from build123d import *

# Parameters (mm, degrees)
ESBO_O1_W                = 514
ESBO_O1_H                = 507
RESSALTO_EXTRUS_O1_DEPTH = 5
ESBO_O2_W                = 5
ESBO_O2_H                = 253.5
RESSALTO_EXTRUS_O2_DEPTH = 10
ESBO_O6_W                = 5
ESBO_O6_H                = 253.5
RESSALTO_EXTRUS_O3_DEPTH = 10
ESBO_O7_W                = 3
ESBO_O7_H                = 253.5
CORTE_EXTRUS_O1_DEPTH    = 10
ESBO_O9_W                = 3
ESBO_O9_H                = 253.5
CORTE_EXTRUS_O3_DEPTH    = 10
ESBO_O10_W               = 514
ESBO_O10_H               = 5
RESSALTO_EXTRUS_O4_DEPTH = 10
ESBO_O15_W               = 512
ESBO_O15_H               = 3
CORTE_EXTRUS_O11_DEPTH   = 10
ESBO_O16_W               = 3
ESBO_O16_H               = 1
CORTE_EXTRUS_O12_DEPTH   = 10
ESBO_O20_R               = 15
RESSALTO_EXTRUS_O5_DEPTH = 10
ESBO_O21_W               = 1
ESBO_O21_H               = 29
CORTE_EXTRUS_O13_DEPTH   = 10


with BuildPart() as part:
    # Esboço1 → Ressalto-extrusão1 (new body)
    with BuildSketch(Plane(origin=(0, 0, 0), x_dir=(1, 0, 0), z_dir=(0, 1, 0))):
        with Locations((159.395426849, -182.414405214)):
            Rectangle(ESBO_O1_W, ESBO_O1_H)
    extrude(amount=RESSALTO_EXTRUS_O1_DEPTH)

    # Esboço2 → Ressalto-extrusão2 (add)
    with BuildSketch(Plane(origin=(0, 5, 0), x_dir=(1, 0, 0), z_dir=(0, 1, 0))):
        with Locations((-95.104573151, -55.664405214)):
            Rectangle(ESBO_O2_W, ESBO_O2_H)
    extrude(amount=RESSALTO_EXTRUS_O2_DEPTH)

    # Esboço6 → Ressalto-extrusão3 (add)
    with BuildSketch(Plane(origin=(0, 5, 0), x_dir=(1, 0, 0), z_dir=(0, 1, 0))):
        with Locations((413.895426849, -55.664405214)):
            Rectangle(ESBO_O6_W, ESBO_O6_H)
    extrude(amount=RESSALTO_EXTRUS_O3_DEPTH)

    # Esboço7 → Corte-extrusão1 (cut)
    with BuildSketch(Plane(origin=(0, 15, 0), x_dir=(1, 0, 0), z_dir=(0, 1, 0))):
        with Locations((-95.104573151, -55.664405214)):
            Rectangle(ESBO_O7_W, ESBO_O7_H)
    extrude(amount=-CORTE_EXTRUS_O1_DEPTH, mode=Mode.SUBTRACT)

    # Esboço9 → Corte-extrusão3 (cut)
    with BuildSketch(Plane(origin=(0, 15, 0), x_dir=(1, 0, 0), z_dir=(0, 1, 0))):
        with Locations((413.895426849, -55.664405214)):
            Rectangle(ESBO_O9_W, ESBO_O9_H)
    extrude(amount=-CORTE_EXTRUS_O3_DEPTH, mode=Mode.SUBTRACT)

    # Esboço10 → Ressalto-extrusão4 (add)
    with BuildSketch(Plane(origin=(0, 5, 0), x_dir=(1, 0, 0), z_dir=(0, 1, 0))):
        with Locations((159.395426849, 68.585594786)):
            Rectangle(ESBO_O10_W, ESBO_O10_H)
    extrude(amount=RESSALTO_EXTRUS_O4_DEPTH)

    # Esboço15 → Corte-extrusão11 (cut)
    with BuildSketch(Plane(origin=(0, 15, 0), x_dir=(1, 0, 0), z_dir=(0, 1, 0))):
        with Locations((159.395426849, 68.585594786)):
            Rectangle(ESBO_O15_W, ESBO_O15_H)
    extrude(amount=-CORTE_EXTRUS_O11_DEPTH, mode=Mode.SUBTRACT)

    # Esboço16 → Corte-extrusão12 (cut)
    with BuildSketch(Plane(origin=(0, 15, 0), x_dir=(1, 0, 0), z_dir=(0, 1, 0))):
        with Locations((413.895426849, 66.585594786)):
            Rectangle(ESBO_O16_W, ESBO_O16_H)
        with Locations((-95.104573151, 66.585594786)):
            Rectangle(ESBO_O16_W, ESBO_O16_H)
    extrude(amount=-CORTE_EXTRUS_O12_DEPTH, mode=Mode.SUBTRACT)

    # Esboço20 → Ressalto-extrusão5 (add)
    with BuildSketch(Plane.XZ):
        with Locations(Location((-47.604573151, 385.914405214, 0), (0, 0, 90))):
            Circle(ESBO_O20_R)
        with Locations(Location((366.395426849, 385.914405214, 0), (0, 0, 90))):
            Circle(ESBO_O20_R)
        with Locations(Location((366.395426849, -21.085594786, 0), (0, 0, 90))):
            Circle(ESBO_O20_R)
        with Locations(Location((-47.604573151, -21.085594786, 0), (0, 0, 90))):
            Circle(ESBO_O20_R)
    extrude(amount=RESSALTO_EXTRUS_O5_DEPTH)

    # Esboço21 → Corte-extrusão13 (cut)
    with BuildSketch(Plane(origin=(0, 15, 0), x_dir=(1, 0, 0), z_dir=(0, 1, 0))):
        with Locations((411.895426849, 51.585594786)):
            Rectangle(ESBO_O21_W, ESBO_O21_H)
        with Locations((415.895426849, 51.585594786)):
            Rectangle(ESBO_O21_W, ESBO_O21_H)
    extrude(amount=-CORTE_EXTRUS_O13_DEPTH, mode=Mode.SUBTRACT)


solid = part.part
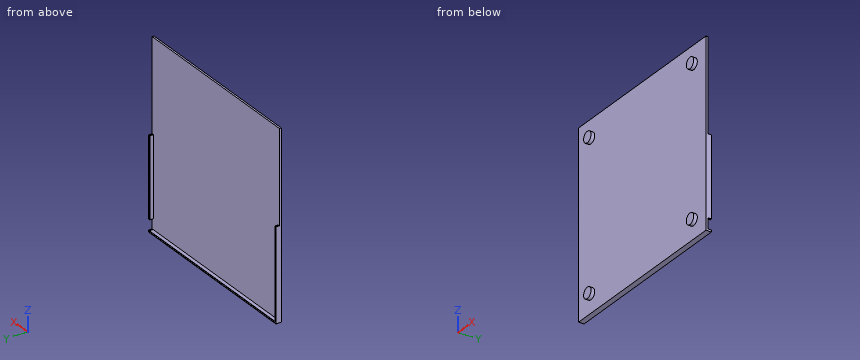
Verification items for the finished model (mm, model axes). Round coordinates to 2 decimals unless told otherwise and drop trailing zeros. Order: outer loops, then holes, each group sorted by start corner. A loop starts at its lowest first (then second) coordinate and runs counter-clockwise, first axis right, second up.
1. Section check D-D on z = 232. Record the cut outline in (x, y), then the cut area to 3 significant figures.
Final values:
outline: (-97.6, 0) - (416.4, 0) - (416.4, 5) - (-97.6, 5) - close
area: 2,570 mm2
2. Section check A-A on x = 321. Record the cut outline in (y, z).
Final values:
outline: (0, -71.09) - (15, -71.09) - (15, -70.09) - (5, -70.09) - (5, -67.09) - (15, -67.09) - (15, -66.09) - (5, -66.09) - (5, 435.91) - (0, 435.91) - close
3. Section check C-C on y = -4.25. Record the cut outline in (x, z).
Final values:
outline: circle Ø30 at (-47.6, -21.09); circle Ø30 at (-47.6, 385.91); circle Ø30 at (366.4, -21.09); circle Ø30 at (366.4, 385.91)
4. Section check B-B on z = 98. Record the cut outline in (x, y).
Final values:
outline: (-97.6, 0) - (416.4, 0) - (416.4, 15) - (415.4, 15) - (415.4, 5) - (412.4, 5) - (412.4, 15) - (411.4, 15) - (411.4, 5) - (-92.6, 5) - (-92.6, 15) - (-93.6, 15) - (-93.6, 5) - (-96.6, 5) - (-96.6, 15) - (-97.6, 15) - close
5. Go/stop test with flat-tipped pins: P1, Ø5, axis at x = 84, z = -19, coming from the +Y side; P2, Ø5, axis at x = 133.5, y = 10.5, coming from the +Z side; P3, Ø0.5, axis at x = -97, y = 9.5, coming from the +Z side. Record where each tip stops, or that it passes through.
Final values:
P1: stops at y = 5
P2: stops at z = -66.09
P3: stops at z = 182.41
6. Thickness scan on L1, parallel to X at y = 11.75, z = 11; L2, parallel to Z at x = 100, y = 13.75; L3, parallel to Y at x = -60.5, z = 132. Record the ranges inside material, lowest first.
Final values:
L1: x = -97.6 to -96.6, -93.6 to -92.6, 411.4 to 412.4, 415.4 to 416.4
L2: z = -71.09 to -70.09, -67.09 to -66.09
L3: y = 0 to 5
